Here's the drawing with two shaded views (mm, measured from the low corner). I have some questions. Give positions to 0.01 mm unless a question says otherwise; leave off trailing zeros. Loops run counter-clockwise (first coordinate to the right, second up) from the corner with the lowest first, then second, coordinate; pieces in that order, holes last. Notation, with made-up numbers: (4, 87) - (17, 87) arc R16 cw to (17, 109) - close; hole circle Ø5 at (49.25, -33.75). An arc over 180 degrees is marked (long way). Write each question's results on one line, items separated by ' | '. Start each with the question number.
1) If I drill on probe 1 along Y at (x, z) = (3.6, 24); probe 2 along Z at (x, y) = (1.85, 20); probe 3 along Y at (x, z) = (1.2, 12.5), over which ranges is the centre line in solid material (lowest first)? Write a range as [from, to].
2) I'm going to push flat-ended pins straight in: pin 1 (1.2 mm diameter, centred on x = 2.5, y = 148, fed in from -Z); pin 2 (2 mm diameter, centred on x = 3.5, z = 14, fed in from +Y); pin 3 (3 mm diameter, centred on y = 130, z = 11, fed in from +X); pin 4 (1.2 mm diameter, centred on x = 2, z = 22.5, fed in from -Y). Where does each tip first touch, or does it pass through?
3) I want a section at B-B, the plane x = 2.9. Write out the boundary of the cut face in (y, z).
4) I want a section at C-C, the plane z = 11. Write out the boundary of the cut face in (x, y), and give its area (3 significant figures).
5) I want a section at A-A, the plane y = 109. Write out the boundary of the cut face in (x, z).
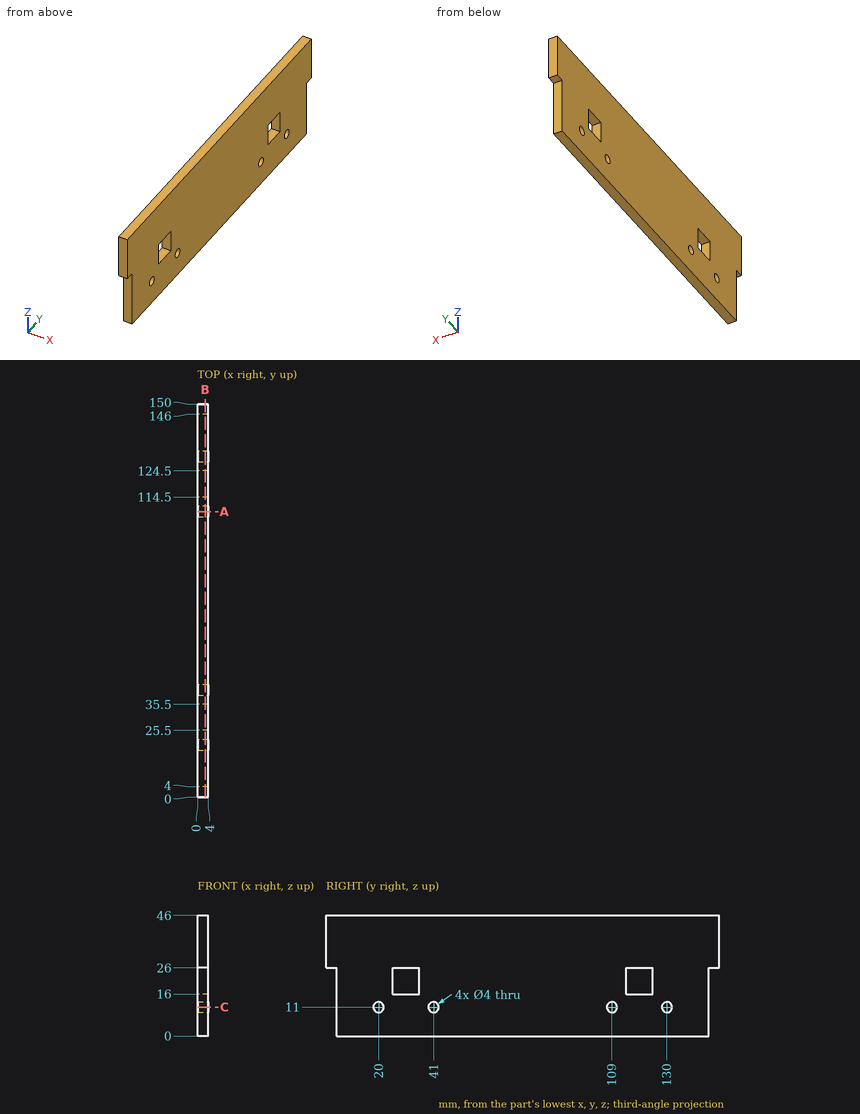
Answers:
1) probe 1: y = [4, 25.5], [35.5, 114.5], [124.5, 146] | probe 2: z = [0, 9], [13, 46] | probe 3: y = [4, 18.68], [21.32, 39.68], [42.32, 107.68], [110.32, 128.68], [131.32, 146]
2) pin 1: stops at z = 26 | pin 2: stops at y = 146 | pin 3: passes through | pin 4: stops at y = 4
3) outline: (0, 26) - (4, 26) - (4, 0) - (146, 0) - (146, 26) - (150, 26) - (150, 46) - (0, 46) - close; hole circle Ø4 at (20, 11); hole (25.5, 16) - (35.5, 16) - (35.5, 26) - (25.5, 26) - close; hole circle Ø4 at (41, 11); hole circle Ø4 at (109, 11); hole (114.5, 16) - (124.5, 16) - (124.5, 26) - (114.5, 26) - close; hole circle Ø4 at (130, 11)
4) outline: (0, 4) - (4, 4) - (4, 18) - (0, 18) - close; (0, 22) - (4, 22) - (4, 39) - (0, 39) - close; (0, 43) - (4, 43) - (4, 107) - (0, 107) - close; (0, 111) - (4, 111) - (4, 128) - (0, 128) - close; (0, 132) - (4, 132) - (4, 146) - (0, 146) - close | area: 504 mm2
5) outline: (0, 0) - (4, 0) - (4, 9) - (0, 9) - close; (0, 13) - (4, 13) - (4, 46) - (0, 46) - close
